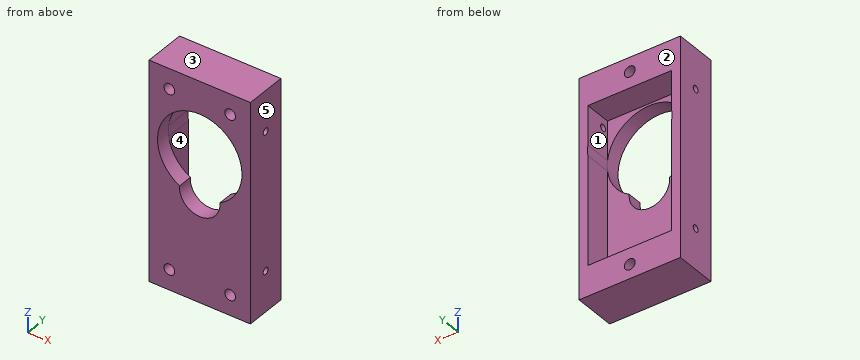
```python
from build123d import *
from build123d.topology import SkipClean

# Parameters (mm, degrees)
SKETCH_1_W          = 15
SKETCH_1_H          = 32.4
SKETCH_1_R          = 0.8
EXTRUDE_1_DEPTH     = 2.2
SKETCH_1_3_R        = 6.25
SKETCH_1_3_R_2      = 3
CUT_EXTRUDE_1_DEPTH = 36.771497033
SKETCH_2_W          = 12.4
SKETCH_2_H          = 4.5
SKETCH_2_R          = 0.8
SKETCH_2_W_2        = 1.3
EXTRUDE_2_DEPTH     = 4
SKETCH_3_R          = 0.8
CUT_EXTRUDE_2_DEPTH = 3
SKETCH_4_R          = 0.5
CUT_EXTRUDE_3_DEPTH = 37.238101496


with BuildPart() as part:
    # Sketch 1 → Extrude 1 (new body)
    with BuildSketch(Plane(origin=(0, 0, 0), x_dir=(1, 0, 0), z_dir=(0, 1, 0))):
        with Locations((7.5, -16.2)):
            Rectangle(SKETCH_1_W, SKETCH_1_H)
        with Locations(Location((3, -3, 0), (0, 0, 270))):
            Circle(SKETCH_1_R, mode=Mode.SUBTRACT)
        with Locations(Location((12, -3, 0), (0, 0, 270))):
            Circle(SKETCH_1_R, mode=Mode.SUBTRACT)
        with Locations(Location((3, -29.4, 0), (0, 0, 270))):
            Circle(SKETCH_1_R, mode=Mode.SUBTRACT)
        with Locations(Location((12, -29.4, 0), (0, 0, 270))):
            Circle(SKETCH_1_R, mode=Mode.SUBTRACT)
    extrude(amount=EXTRUDE_1_DEPTH)

    # Sketch 1_3 → Cut-Extrude 1 (cut, through all)
    with BuildSketch(Plane(origin=(0, 0, 0), x_dir=(1, 0, 0), z_dir=(0, 1, 0))):
        with Locations((7.5, -21.35)):
            Circle(SKETCH_1_3_R)
        with Locations((7.5, -15.6)):
            Circle(SKETCH_1_3_R_2)
    extrude(amount=CUT_EXTRUDE_1_DEPTH, mode=Mode.SUBTRACT)

    # Sketch 2 → Extrude 2 (add)
    # profile 1 of 12: a face of its own
    with SkipClean():  # the faces are left unmerged after this step: merging them gives an invalid solid
        with BuildSketch(Plane(origin=(0, 2.2, 0), x_dir=(1, 0, 0), z_dir=(0, 1, 0))):
            with Locations((7.5, -2.25)):
                Rectangle(SKETCH_2_W, SKETCH_2_H)
            with Locations(Location((3, -3, 0), (0, 0, 270))):
                Circle(SKETCH_2_R, mode=Mode.SUBTRACT)
            with Locations(Location((12, -3, 0), (0, 0, 270))):
                Circle(SKETCH_2_R, mode=Mode.SUBTRACT)
        # profile 2 of 12: a face of its own
        with BuildSketch(Plane(origin=(0, 2.2, 0), x_dir=(1, 0, 0), z_dir=(0, 1, 0))):
            with Locations((0.65, -2.25)):
                Rectangle(SKETCH_2_W_2, SKETCH_2_H)
        # profile 3 of 12: a face of its own
        with BuildSketch(Plane(origin=(0, 2.2, 0), x_dir=(1, 0, 0), z_dir=(0, 1, 0))):
            with Locations((14.35, -2.25)):
                Rectangle(SKETCH_2_W_2, SKETCH_2_H)
        # profile 4 of 12: a face of its own
        with BuildSketch(Plane(origin=(0, 2.2, 0), x_dir=(1, 0, 0), z_dir=(0, 1, 0))):
            with Locations((7.5, -30.15)):
                Rectangle(SKETCH_2_W, SKETCH_2_H)
            with Locations(Location((3, -29.4, 0), (0, 0, 270))):
                Circle(SKETCH_2_R, mode=Mode.SUBTRACT)
            with Locations(Location((12, -29.4, 0), (0, 0, 270))):
                Circle(SKETCH_2_R, mode=Mode.SUBTRACT)
        # profile 5 of 12: a face of its own
        with BuildSketch(Plane(origin=(0, 2.2, 0), x_dir=(1, 0, 0), z_dir=(0, 1, 0))):
            with Locations((0.65, -30.15)):
                Rectangle(SKETCH_2_W_2, SKETCH_2_H)
        # profile 6 of 12: a face of its own
        with BuildSketch(Plane(origin=(0, 2.2, 0), x_dir=(1, 0, 0), z_dir=(0, 1, 0))):
            with Locations((14.35, -30.15)):
                Rectangle(SKETCH_2_W_2, SKETCH_2_H)
        # profile 7 of 12: a face of its own
        with BuildSketch(Plane(origin=(0, 2.2, 0), x_dir=(1, 0, 0), z_dir=(0, 1, 0))):
            with Locations(Location((3, -3, 0), (0, 0, 270))):
                Circle(SKETCH_2_R)
        # profile 8 of 12: a face of its own
        with BuildSketch(Plane(origin=(0, 2.2, 0), x_dir=(1, 0, 0), z_dir=(0, 1, 0))):
            with Locations(Location((12, -3, 0), (0, 0, 270))):
                Circle(SKETCH_2_R)
        # profile 9 of 12: a face of its own
        with BuildSketch(Plane(origin=(0, 2.2, 0), x_dir=(1, 0, 0), z_dir=(0, 1, 0))):
            with Locations(Location((3, -29.4, 0), (0, 0, 270))):
                Circle(SKETCH_2_R)
        # profile 10 of 12: a face of its own
        with BuildSketch(Plane(origin=(0, 2.2, 0), x_dir=(1, 0, 0), z_dir=(0, 1, 0))):
            with Locations(Location((12, -29.4, 0), (0, 0, 270))):
                Circle(SKETCH_2_R)
        # profile 11 of 12: a face of its own
        with BuildSketch(Plane(origin=(0, 2.2, 0), x_dir=(1, 0, 0), z_dir=(0, 1, 0))):
            with BuildLine():
                Line((13.7, -27.9), (15, -27.9))
                Line((15, -27.9), (15, -4.5))
                Line((15, -4.5), (13.7, -4.5))
                Line((13.7, -4.5), (13.7, -20.561013308))
                ThreePointArc((13.7, -20.561013308), (13.75, -21.35), (13.7, -22.138986692))
                Line((13.7, -22.138986692), (13.7, -27.9))
            make_face()
        # profile 12 of 12: a face of its own
        with BuildSketch(Plane(origin=(0, 2.2, 0), x_dir=(1, 0, 0), z_dir=(0, 1, 0))):
            with BuildLine():
                Line((0, -27.9), (1.3, -27.9))
                Line((1.3, -27.9), (1.3, -22.138986692))
                ThreePointArc((1.3, -22.138986692), (1.25, -21.35), (1.3, -20.561013308))
                Line((1.3, -20.561013308), (1.3, -4.5))
                Line((1.3, -4.5), (0, -4.5))
                Line((0, -4.5), (0, -27.9))
            make_face()
        extrude(amount=EXTRUDE_2_DEPTH)

    # Sketch 3 → Cut-Extrude 2 (cut)
    with SkipClean():  # the faces are left unmerged after this step: merging them gives an invalid solid
        with BuildSketch(Plane(origin=(0, 6.2, 0), x_dir=(1, 0, 0), z_dir=(0, 1, 0))):
            with Locations(Location((7.5, -30.3, 0), (0, 0, 180))):
                Circle(SKETCH_3_R)
            with Locations(Location((7.5, -2.1, 0), (0, 0, 180))):
                Circle(SKETCH_3_R)
        extrude(amount=-CUT_EXTRUDE_2_DEPTH, mode=Mode.SUBTRACT)

    # Sketch 4 → Cut-Extrude 3 (cut, through all)
    with SkipClean():  # the faces are left unmerged after this step: merging them gives an invalid solid
        with BuildSketch(Plane.ZY):
            with Locations((6, 3.1)):
                Circle(SKETCH_4_R)
            with Locations((26.4, 3.1)):
                Circle(SKETCH_4_R)
        extrude(amount=-CUT_EXTRUDE_3_DEPTH, mode=Mode.SUBTRACT)


solid = part.part
```
The model under review builds one solid part; all positions refer to its coordinate system, in mm. Face numbers are marked on the shaded views. A direction names the side the tool comes from. Give positions to 0.01 mm unless a question says otherwise; leave off trailing zeros. Write each loop counter-clockwise with the first axis right and the second up, starting at its lowest first coordinate (ties: lowest second). Pieces come first, ordered by that corner, then holes.
(1) Consider section D-D, the plane z = 5. Give the boundary of the cut face in (x, y), and give its area (3 significant figures).
(2) Consider section C-C, the plane z = 21.35. Give the boundary of the cut face in (x, y), and give its area (3 significant figures).
(3) Tool access review of the marked faces 4 and 5: name each direction out of +Z, -Z, +X, -X, +Y, -Y from which nothing blocks a thin tool from reaching the whole face with its end or side.
(4) Consider section B-B, the plane y = 4. Give the boundary of the cut face in (x, z), and give its area (3 significant figures).
(5) For P1, Ø2, axis at x = 7.5, z = 30.3, coming from the +Y side; P2, Ø7.5, axis at x = 7.5, z = 21.35, coming from the -Y side; P3, Ø0.5, axis at x = 2.5, z = 29.5, coming from the -Y side; P4, Ø0.5, axis at x = 7.5, z = 2, coming from the +Y side, all flat-tipped, find the tip position at first contact; note any pin that passes through.
(6) Consider section A-A, the plane x = 7.5. Give the boundary of the cut face in (y, z), and give its area (3 significant figures).
(7) The part is to be moulded in two halves that separate along Z. For the marked faces 1, 2 and 3, say which applies: released by +Z, released by -Z, zero draft, split by the parting line, or undercut.
(8) To check wall thickness, follow L1, parallel to X at y = 0.6, z = 29.4; L2, parallel to Z at x = 7.5, y = 4.85; L3, parallel to X at y = 3.25, z = 14. State the ranges of each line that lie inside material, in increasing order.
Returned:
1. outline: (0, 0) - (15, 0) - (15, 6.2) - (13.7, 6.2) - (13.7, 2.2) - (1.3, 2.2) - (1.3, 6.2) - (0, 6.2) - close
1. area: 43.4 mm2
2. outline: (0, 0) - (1.25, 0) - (1.25, 6.2) - (0, 6.2) - close; (13.75, 0) - (15, 0) - (15, 6.2) - (13.75, 6.2) - close
2. area: 15.5 mm2
3. face 4: +Y
3. face 5: +Z, -Z, +X, +Y, -Y
4. outline: (0, 0) - (15, 0) - (15, 32.4) - (0, 32.4) - close; hole (1.3, 4.5) - (13.7, 4.5) - (13.7, 20.56) arc R6.25 ccw to (13.7, 22.14) - (13.7, 27.9) - (1.3, 27.9) - (1.3, 22.14) arc R6.25 ccw to (1.3, 20.56) - close; hole circle Ø1.6 at (7.5, 2.1); hole circle Ø1.6 at (7.5, 30.3)
4. area: 192 mm2
5. P1: stops at y = 6.2
5. P2: passes through
5. P3: stops at y = 2.2
5. P4: stops at y = 3.2
6. outline: (0, 0) - (6.2, 0) - (6.2, 1.3) - (3.2, 1.3) - (3.2, 2.9) - (6.2, 2.9) - (6.2, 4.5) - (2.2, 4.5) - (2.2, 12.6) - (0, 12.6) - close; (0, 27.6) - (2.2, 27.6) - (2.2, 27.9) - (6.2, 27.9) - (6.2, 29.5) - (3.2, 29.5) - (3.2, 31.1) - (6.2, 31.1) - (6.2, 32.4) - (0, 32.4) - close
6. area: 64.7 mm2
7. face 1: undercut
7. face 2: zero draft
7. face 3: released by +Z
8. L1: x = 0 to 2.2, 3.8 to 11.2, 12.8 to 15
8. L2: z = 0 to 1.3, 2.9 to 4.5, 27.9 to 29.5, 31.1 to 32.4
8. L3: x = 0 to 1.3, 13.7 to 15
